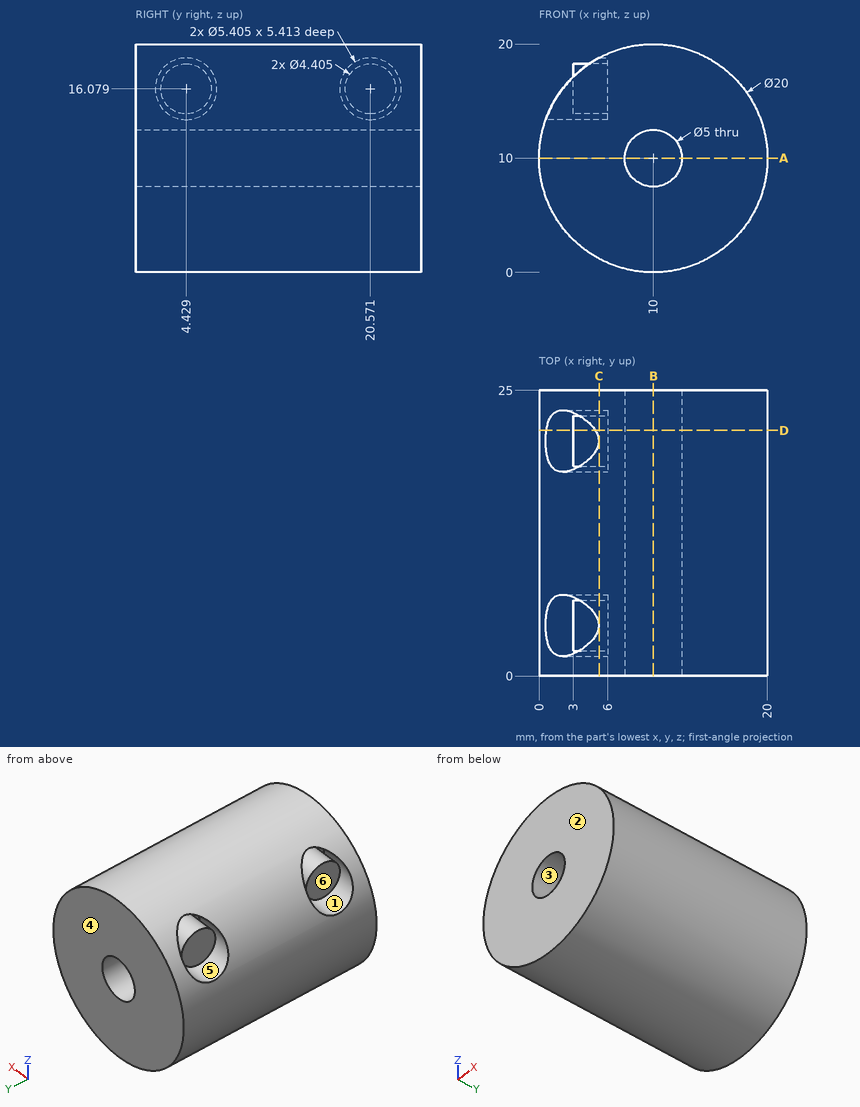
Geometry check sheet. Reference: drawing and pictorial views, mm from the part's lowest x, y, z. A direction names the side the tool comes from. Round coordinates to 2 decimals unless told otherwise and drop trailing zeros. Loops run counter-clockwise (first coordinate to the right, second up) from the corner with the lowest first, then second, coordinate; pieces in that order, holes last. Notation, with made-up numbers: (-32, -17) - (-10, -17) arc R23 ccw to (-10, 1) - close; hole circle Ø7 at (-30, 37). An arc over 180 degrees is marked (long way). Answer in a Markdown table with one row per item. Add a question column.
Q1. Section check D-D on y = 21.5. Enter the section's corners in (x, z) (1 decimal), plus the area to 3 significant figures.
Q2. Release check for a two-part mould opening along Y. For the marked faces 1, 2, 3 and 4 record: pulls with the +Y half, pulls with the -Y half, needs draft (parallel to the pull), parting line crosses it, or undercut.
Q3. Section check A-A on z = 10. Enter the section's corners in (x, y).
Q4. Material ranges on line 1 (X direction, y = 17.25, z = 10); line 2 (Y direction, x = 4.75, z = 16.5); line 3 (Z direction, x = 5.25, y = 5.5) (1 decimal), recorded low to high.
Q5. Section check B-B on x = 10. Enter the section's corners in (y, z), plus the area to 3 significant figures.
Q6. Tool access check on the marked faces 5 and 6. Record the directions out of +Z, -Z, +X, -X, +Y, -Y that give a thin tool (end or side, any length) a straight path to the whole face; none if there is none.
Q7. Gauge pin test, flat ends, axial feed: pin 1 (12 mm diameter, centred on y = 19, z = 3, fed in from +X); pin 2 (6 mm diameter, centred on y = 10, z = 17, fed in from +X) (1 decimal); pin 3 (1.5 mm diameter, centred on x = 15, y = 14.5, fed in from -Z); pin 4 (4 mm diameter, centred on x = 9, y = 14, fed in from -Z). Record the tip position at first contact, or that the pin passes through.
Q8. Section check C-C on x = 5.25. Enter the section's corners in (y, z) (1 decimal).
Found:
| question | item | result |
|---|---|---|
| 1 | outline | (0.6, 13.5) arc R10 ccw (long way) to (4.9, 18.6) - (6, 18.6) - (6, 18.1) - (3, 18.1) - (3, 14.1) - (6, 14.1) - (6, 13.5) - close; hole circle Ø5 at (10, 10) |
| 1 | area | 288 mm² |
| 2 | face 1 | undercut |
| 2 | face 2 | pulls with the -Y half |
| 2 | face 3 | needs draft |
| 2 | face 4 | pulls with the +Y half |
| 3 | outline | (0, 0) - (7.5, 0) - (7.5, 25) - (0, 25) - close; (12.5, 0) - (20, 0) - (20, 25) - (12.5, 25) - close |
| 4 | line 1 | x = 0 to 7.5, 12.5 to 20 |
| 4 | line 2 | y = 0 to 1.76, 2.27 to 6.59, 7.1 to 17.9, 18.41 to 22.73, 23.24 to 25 |
| 4 | line 3 | z = 1.2 to 13.6, 14.2 to 18, 18.6 to 18.8 |
| 5 | outline | (0, 0) - (25, 0) - (25, 7.5) - (0, 7.5) - close; (0, 12.5) - (25, 12.5) - (25, 20) - (0, 20) - close |
| 5 | area | 375 mm² |
| 6 | face 5 | -X |
| 6 | face 6 | +Z, -X |
| 7 | pin 1 | stops at x = 19.95 |
| 7 | pin 2 | stops at x = 19.2 |
| 7 | pin 3 | stops at z = 0.95 |
| 7 | pin 4 | stops at z = 0 |
| 8 | outline | (0, 1.2) - (25, 1.2) - (25, 18.8) - (0, 18.8) - close; circle Ø4.4 at (4.4, 16.1); circle Ø4.4 at (20.6, 16.1); hole circle Ø5.4 at (4.4, 16.1); hole circle Ø5.4 at (20.6, 16.1) |
